Check sheet for the modelled part. Datum: model origin and axes. Units: mm. Face numbers are marked on the shaded views. A direction names the side the tool comes from. Round coordinates to 2 decimals unless told otherwise and drop trailing zeros. Order: outer loops, then holes, each group sorted by start corner. A loop starts at its lowest first (then second) coordinate and runs counter-clockwise, first axis right, second up. Notation, with made-up numbers: (61.5, 58) -> (115.5, 58) arc R25 cw to (115.5, 97) -> close; hole circle Ø5 at (6, 63.25). An arc over 180 degrees is marked (long way). Answer in a Markdown table with one row per item.
```python
from build123d import *

# Parameters (mm, degrees)
SKETCH1_W           = 20
SKETCH1_H           = 25
BOSS_EXTRUDE1_DEPTH = 5
SKETCH2_R           = 2.5
BOSS_EXTRUDE2_DEPTH = 3.5
CUT_EXTRUDE1_DEPTH  = 23.5
CUT_EXTRUDE2_DEPTH  = 33.5


with BuildPart() as part:
    # Sketch1 → Boss-Extrude1 (new body)
    with BuildSketch(Plane.XY):
        with Locations((10, 12.5)):
            Rectangle(SKETCH1_W, SKETCH1_H)
    extrude(amount=BOSS_EXTRUDE1_DEPTH)

    # Sketch2 → Boss-Extrude2 (add)
    with BuildSketch(Plane.XY.offset(5)):
        with Locations(Location((4, 19, 0), (0, 0, 180))):
            Circle(SKETCH2_R)
        with Locations(Location((16, 19, 0), (0, 0, 180))):
            Circle(SKETCH2_R)
        with Locations(Location((16, 6, 0), (0, 0, 180))):
            Circle(SKETCH2_R)
        with Locations(Location((4, 6, 0), (0, 0, 180))):
            Circle(SKETCH2_R)
    extrude(amount=BOSS_EXTRUDE2_DEPTH)

    # Sketch3 → Cut-Extrude1 (cut)
    with BuildSketch(Plane(origin=(20, 0, 0), x_dir=(0, 0, -1), z_dir=(1, 0, 0))):
        Polygon((0, 22), (-2.5, 12.5), (0, 12.5), align=None)
        Polygon((0, 12.5), (-2.5, 12.5), (0, 3), align=None)
    extrude(amount=-CUT_EXTRUDE1_DEPTH, mode=Mode.SUBTRACT)

    # Sketch4 → Cut-Extrude2 (cut)
    with BuildSketch(Plane(origin=(0, 0, 0), x_dir=(-1, 0, 0), z_dir=(0, -1, 0))):
        Polygon((0, 0), (-10, -2.5), (-20, 0), align=None)
    extrude(amount=-CUT_EXTRUDE2_DEPTH, mode=Mode.SUBTRACT)


solid = part.part
```
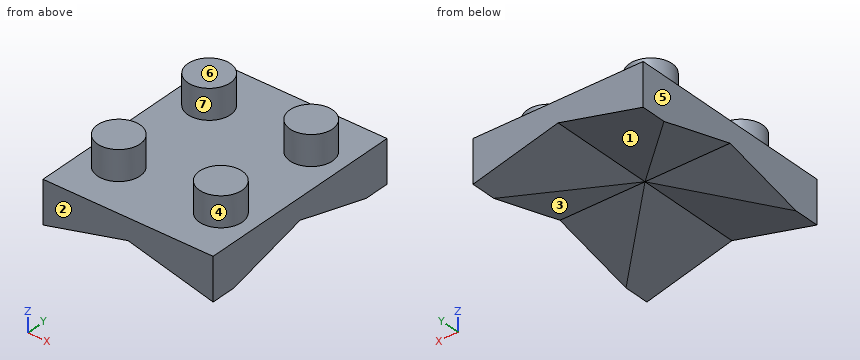
(1) Tool access check on the marked faces 1, 2, 3 and 4. Record the directions out of +Z, -Z, +X, -X, +Y, -Y that give a thin tool (end or side, any length) a straight path to the whole face; none if there is none.
Solutions:
| item | result |
|---|---|
| face 1 | -Z, +Y, -Y |
| face 2 | +Z, -Z, +X, -X, -Y |
| face 3 | -Z, +X, -X |
| face 4 | +Z |
(2) Depth check by flat-ended pin: pin 1 Ø4 at (x, y) = (14.5, 22.5) entering from -Z (3 decimals); pin 2 Ø1.5 at (x, y) = (3.5, 9) entering from -Z. Enter the tip coordinate at first touch or a pass-through.
Solutions:
| item | result |
|---|---|
| pin 1 | z = 0.875 |
| pin 2 | z = 1.38 |
(3) Scan lines: probe 1 along Y at (x, z) = (15.5, 7); probe 2 along Z at (x, y) = (13.25, 5); probe 3 along Y at (x, z) = (4.25, 7.5). Record each from-to range of solid material in increasing order. Write a range as from..to.
Solutions:
| item | result |
|---|---|
| probe 1 | 3.55..8.45, 16.55..21.45 |
| probe 2 | 1.69..5 |
| probe 3 | 3.51..8.49, 16.51..21.49 |
(4) Section check C-C on y = 23.25. Record the boundary of the cut face in (x, z).
Solutions:
| item | result |
|---|---|
| outline | (0, 0) -> (10, 2.5) -> (20, 0) -> (20, 5) -> (0, 5) -> close |
(5) Draft check along X on the marked faces 5, 6 and 7. Enter one of: pulls with the +X half, pulls with the -X half, needs draft (parallel to the pull), parting line crosses it, or undercut.
Solutions:
| item | result |
|---|---|
| face 5 | pulls with the -X half |
| face 6 | needs draft |
| face 7 | undercut |
(6) Section check B-B on x = 4. Record the boundary of the cut face in (y, z), plus the area to 3 significant figures.
Solutions:
| item | result |
|---|---|
| outline | (0, 1) -> (6.8, 1) -> (12.5, 2.5) -> (18.2, 1) -> (25, 1) -> (25, 5) -> (21.5, 5) -> (21.5, 8.5) -> (16.5, 8.5) -> (16.5, 5) -> (8.5, 5) -> (8.5, 8.5) -> (3.5, 8.5) -> (3.5, 5) -> (0, 5) -> close |
| area | 126 mm^2 |
(7) Section check A-A on z = 1. Record the boundary of the cut face in (x, y), plus the area to 3 significant figures.
Solutions:
| item | result |
|---|---|
| outline | (0, 0) -> (4, 0) -> (4, 6.8) -> (0, 6.8) -> close; (0, 18.2) -> (4, 18.2) -> (4, 25) -> (0, 25) -> close; (16, 0) -> (20, 0) -> (20, 6.8) -> (16, 6.8) -> close; (16, 18.2) -> (20, 18.2) -> (20, 25) -> (16, 25) -> close |
| area | 109 mm^2 |
(8) Section check D-D on z = 5.75. Record the boundary of the cut face in (x, y).
Solutions:
| item | result |
|---|---|
| outline | circle Ø5 at (4, 6); circle Ø5 at (4, 19); circle Ø5 at (16, 6); circle Ø5 at (16, 19) |
